from build123d import *

# Parameters (mm, degrees)
F0_R     = 41.4149264742
F0_R_2   = 27.9229275401
F1_DEPTH = 45
F3_DEPTH = 14
F5_DEPTH = 5


with BuildPart() as f1:
    # F0 (on Top) → F1 (new body)
    with BuildSketch(Plane.XY):
        with Locations((32.4097648263, 0)):
            Circle(F0_R)
        with Locations((32.4097648263, 0)):
            Circle(F0_R_2, mode=Mode.SUBTRACT)
    extrude(amount=F1_DEPTH)

    # F2 (on face) → F3 (join)
    with BuildSketch(Plane(origin=(0, 0, 0), x_dir=(1, 0, 0), z_dir=(0, 0, -1))):
        with BuildLine():
            Line((-52.9098688311, -35.7817081915), (11.5563360013, -35.7817081915))
            ThreePointArc((11.5563360013, -35.7817081915), (-9.0051616479, 0), (11.5563360013, 35.7817081915))
            Line((11.5563360013, 35.7817081915), (-52.9098688311, 35.7817081915))
            Line((-52.9098688311, 35.7817081915), (-52.9098688311, -35.7817081915))
        make_face()
    extrude(amount=-F3_DEPTH)

    # F4 (on Front) → F5 (join, symmetric)
    with BuildSketch(Plane.XZ):
        Polygon((-6.9038993679, 43.7489598989), (-47.6915575564, 12.0960362256), (-6.9038993679, 12.0960362256), align=None)
    extrude(amount=F5_DEPTH, both=True)


solid = f1.part
Can you work these out from the model? Positions are in its coordinate system, mm. A direction names the side the tool comes from. Round coordinates to 2 decimals unless told otherwise and drop trailing zeros. Order: outer loops, then holes, each group sorted by start corner. A loop starts at its lowest first (then second) coordinate and runs counter-clockwise, first axis right, second up. Notation, with made-up numbers: (42.5, 74) -> (71.5, 74) arc R22 cw to (71.5, 98) -> close; hole circle Ø5 at (-36, -19). An arc over 180 degrees is marked (long way). Write each question's results on one line, items separated by ' | '. Start each with the question number.
Item 1: If we section it at D-D, the plane x = 15: Write out the boundary of the cut face in (y, z), then the cut area to 3 significant figures.
Item 2: Which directions (+Z, -Z, +X, -X, +Y, -Y) give clear straight access to the entire face, cutting with the end or side of a thin tool? Please do faces 5 (the flat face through (-20, -35.782, 7)), 6 (the flat face through (-28, -8, 14)), 7 (the flat face through (-26.71, -0.07, 28.38)), 8 (the flat face through (-19, 5, 22)), 9 (the flat face through (-19, -5, 22)).
Item 3: Will these pins go through, and if not, where does the flat tip stop? pin 1 (2 mm diameter, centred on x = 3.5, z = 31.5, fed in from -Y); pin 2 (8.5 mm diameter, centred on x = -27.5, z = 30, fed in from -Y); pin 3 (8.5 mm diameter, centred on x = -18, z = 30.5, fed in from +Y).
Item 4: If we section it at B-B, the plane x = 48: Write out the boundary of the cut face in (y, z), then the cut area to 3 significant figures.
Item 5: If we section it at C-C, the plane z = 11: Write out the boundary of the cut face in (x, y), then the cut area to 3 significant figures.
Item 6: If we section it at A-A, the plane y = 0: Write out the boundary of the cut face in (x, z), then the cut area to 3 significant figures.
Item 7: Thinking about a two-plate mould opening in Y: for faces 1 (the cylindrical face through (71.912, 12.44, 22.185)), 2 (the flat face through (-21, 35.782, 7)), 3 (the flat face through (-52.91, -1, 7)), 4 (the cylindrical face through (58.2, -10.7, 22.2)), which applies, +Y half, -Y half, draft (parallel to the pull), parting line (faces both ways), or undercut?
Item 8: Please list where these lines run through material, in increasing order: L1, parallel to Y at x = -13, z = 37; L2, parallel to X at y = 12, z = 22.5; L3, parallel to X at y = 11, z = 19.
Results:
1) outline: (-37.58, 0) -> (-21.83, 0) -> (-21.83, 45) -> (-37.58, 45) -> close; (21.83, 0) -> (37.58, 0) -> (37.58, 45) -> (21.83, 45) -> close | area: 1,420 mm2
2) face 5: +Z, -Z, -X, -Y | face 6: +Z, -X | face 7: +Z, -X, +Y, -Y | face 8: +Z, -X, +Y | face 9: +Z, -X, -Y
3) pin 1: stops at y = -30.6 | pin 2: stops at y = -5 | pin 3: stops at y = 5
4) outline: (-38.37, 0) -> (-23.17, 0) -> (-23.17, 45) -> (-38.37, 45) -> close; (23.17, 0) -> (38.37, 0) -> (38.37, 45) -> (23.17, 45) -> close | area: 1,370 mm2
5) outline: (-52.91, -35.78) -> (11.56, -35.78) arc R41.41 ccw (long way) to (11.56, 35.78) -> (-52.91, 35.78) -> close; hole circle Ø55.85 at (32.41, 0) | area: 6,510 mm2
6) outline: (-52.91, 0) -> (4.49, 0) -> (4.49, 45) -> (-9.01, 45) -> (-9.01, 42.12) -> (-45.24, 14) -> (-52.91, 14) -> close; (60.33, 0) -> (73.82, 0) -> (73.82, 45) -> (60.33, 45) -> close | area: 2,340 mm2
7) face 1: parting line | face 2: +Y half | face 3: draft | face 4: undercut
8) L1: y = -5 to 5 | L2: x = -7.23 to 7.2, 57.62 to 72.05 | L3: x = -7.52 to 6.74, 58.07 to 72.34
